from build123d import *

# Parameters (mm, degrees)
FILLET1_R = 1


with BuildPart() as part:
    # Sketch1 → Revolve1 (revolve)
    with BuildSketch(Plane(origin=(0, 0, 0), x_dir=(0, 0, -1), z_dir=(1, 0, 0))):
        Polygon((2.1, 6), (4.25, 6), (4.25, 12), (8.25, 12), (10.5, 0), (2.1, 0), align=None)
    revolve(axis=Axis((0, 0, 0), (0, 1, 0)))

    # Fillet1
    fillet1_edges = [part.edges().sort_by_distance(p)[0] for p in [
        (0, 12, 8.25),
        (0, 12, 4.25),
    ]]
    fillet(fillet1_edges, radius=FILLET1_R)


solid = part.part
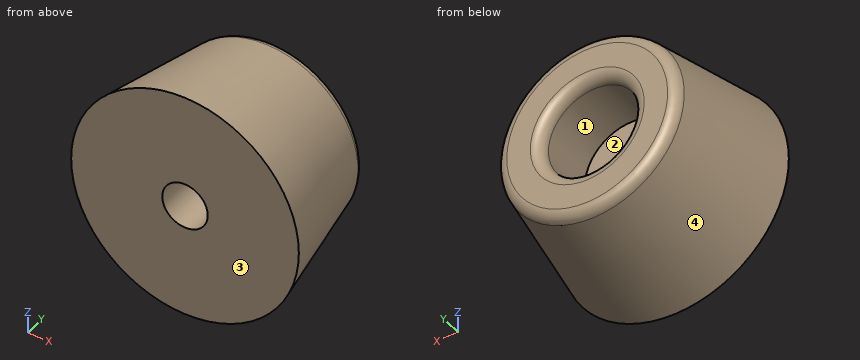
Read the model definition and answer for the solid it produces. Units are mm, in the model's axes. Face numbers are marked on the shaded views. Coordinates: 2 decimals unless noted, no trailing zeros. Order: outer loops, then holes, each group sorted by start corner. A loop starts at its lowest first (then second) coordinate and runs counter-clockwise, first axis right, second up. Notation, with made-up numbers: M 11,13.5 L 51,13.5 A23 ccw 51,25.5 Z; hole C 70.5,88.5 d2. An arc over 180 degrees is marked long. Put each result on its own line as item: value. Start each with the question number.
Item 1: The mould has two halves that part along Z. Classify the marked faces 1, 2, 3 and 4: +Z half, -Z half, draft (parallel to the pull), parting line (faces both ways), or undercut.
Item 2: Given pin 1 Ø10 at (x, z) = (8, -1) entering from -Y; pin 2 Ø2 at (y, z) = (8.5, 0.5) entering from +X; pin 3 Ø4 at (x, y) = (-5.5, 5) entering from +Z; pin 4 Ø2 at (x, y) = (-4.5, 11) entering from -Z, each flat-ended and moving along its own axis, determine where each tip first touches the part or whether it passes through.
Item 3: Consider probe 1 along Y at (x, z) = (1, -3.5); probe 2 along Z at (x, y) = (0, 2.25); probe 3 along X at (y, z) = (6.75, -5.5). Determine where each line is inside the solid, lowest interval first. Write a range as [from, to].
Item 4: Section B-B, the plane z = 0 is taken. Determine the outline of the cut face in (x, y).
Item 5: Section D-D, the plane y = 3.25 is taken. Determine the outline of the cut face in (x, z).
Item 6: Section A-A, the plane x = 0 is taken. Determine the outline of the cut face in (y, z), plus the area to 3 significant figures.
Item 7: Section C-C, the plane y = 7.25 is taken. Determine the outline of the cut face in (x, z).
Computed:
1. face 1: undercut
1. face 2: undercut
1. face 3: draft
1. face 4: parting line
2. pin 1: stops at y = 0
2. pin 2: stops at x = 9.09
2. pin 3: stops at z = 8.99
2. pin 4: stops at z = -7.72
3. probe 1: y = [0, 6]
3. probe 2: z = [-10.08, -2.1], [2.1, 10.08]
3. probe 3: x = [-7.42, 7.42]
4. outline: M -10.5,0 L -2.1,0 L -2.1,6 L -4.25,6 L -4.25,11 A1 ccw -5.25,12 L -7.42,12 A1 ccw -8.4,11.18 Z; M 2.1,0 L 10.5,0 L 8.4,11.18 A1 ccw 7.42,12 L 5.25,12 A1 ccw 4.25,11 L 4.25,6 L 2.1,6 Z
5. outline: C 0,0 d19.78; hole C 0,0 d4.2
6. outline: M 0,-10.5 L 11.18,-8.4 A1 ccw 12,-7.42 L 12,-5.25 A1 ccw 11,-4.25 L 6,-4.25 L 6,-2.1 L 0,-2.1 Z; M 0,2.1 L 6,2.1 L 6,4.25 L 11,4.25 A1 ccw 12,5.25 L 12,7.42 A1 ccw 11.18,8.4 L 0,10.5 Z
6. area: 148 mm2
7. outline: C 0,0 d18.28; hole C 0,0 d8.5
